```python
from build123d import *

# Parameters (mm, degrees)
SKETCH_1_W                  = 60
SKETCH_1_H                  = 45
SKETCH_1_R                  = 2.5
SKETCH_1_R_2                = 12
EXTRUDE_1_DEPTH             = 8
CHAMFER_1_SIZE              = 1
SKETCH_2_R                  = 4
CUT_EXTRUDE_1_DEPTH         = 6
SKETCH_3_R                  = 1.25
CUT_EXTRUDE_2_DEPTH         = 39.34383914
HOLE_WIZARD_2_D             = 6.2
HOLE_WIZARD_2_CSINK_D       = 13.2
HOLE_WIZARD_2_CSINK_ANGLE   = 90
HOLE_WIZARD_2_2_D           = 3.1
HOLE_WIZARD_2_2_CSINK_D     = 6.2
HOLE_WIZARD_2_2_CSINK_ANGLE = 90


with BuildPart() as part:
    # 草图1 → 凸台-拉伸1 (new body)
    with BuildSketch(Plane(origin=(0, 0, 0), x_dir=(1, 0, 0), z_dir=(0, 1, 0))):
        Rectangle(SKETCH_1_W, SKETCH_1_H)
        with Locations(Location((-20, -12.5, 0), (0, 0, 270))):
            Circle(SKETCH_1_R, mode=Mode.SUBTRACT)
        with Locations(Location((20, -12.5, 0), (0, 0, 90))):
            Circle(SKETCH_1_R, mode=Mode.SUBTRACT)
        with Locations(Location((0, -5, 0), (0, 0, 270))):
            Circle(SKETCH_1_R_2, mode=Mode.SUBTRACT)
    extrude(amount=EXTRUDE_1_DEPTH)

    # 倒角1
    chamfer_1_edges = [part.edges().sort_by_distance(p)[0] for p in [
        (0, 8, -22.5),
        (0, 0, -22.5),
    ]]
    chamfer(chamfer_1_edges, length=CHAMFER_1_SIZE)

    # 草图2 → 切除-拉伸1 (cut)
    with BuildSketch(Plane(origin=(0, 8, 0), x_dir=(1, 0, 0), z_dir=(0, 1, 0))):
        with Locations(Location((-19.5, 14.5, 0), (0, 0, 270))):
            Circle(SKETCH_2_R)
        with Locations(Location((19.5, 14.5, 0), (0, 0, 90))):
            Circle(SKETCH_2_R)
    extrude(amount=-CUT_EXTRUDE_1_DEPTH, mode=Mode.SUBTRACT)

    # 草图3 → 切除-拉伸2 (cut, through all)
    with BuildSketch(Plane(origin=(0, 0, 0), x_dir=(-1, 0, 0), z_dir=(0, -1, 0))):
        with Locations(Location((13, -18, 0), (0, 0, 90))):
            Circle(SKETCH_3_R)
        with Locations(Location((-13, -18, 0), (0, 0, 270))):
            Circle(SKETCH_3_R)
        with Locations(Location((13, 8, 0), (0, 0, 90))):
            Circle(SKETCH_3_R)
        with Locations(Location((-13, 8, 0), (0, 0, 270))):
            Circle(SKETCH_3_R)
    extrude(amount=-CUT_EXTRUDE_2_DEPTH, mode=Mode.SUBTRACT)

    # Hole Wizard 2 (through all)
    with Locations(Plane(origin=(20, 0, 12.5), x_dir=(0, 0, -1), z_dir=(0, -1, 0))):
        with Locations((0, 0), (0, -40)):
            CounterSinkHole(HOLE_WIZARD_2_D / 2, HOLE_WIZARD_2_CSINK_D / 2, counter_sink_angle=HOLE_WIZARD_2_CSINK_ANGLE)

    # Hole Wizard 2 2 (through all)
    with Locations(Plane(origin=(-13, 8, -8), x_dir=(0, 0, 1), z_dir=(0, 1, 0))):
        with Locations((0, 0), (26, 0), (26, 26), (0, 26)):
            CounterSinkHole(HOLE_WIZARD_2_2_D / 2, HOLE_WIZARD_2_2_CSINK_D / 2, counter_sink_angle=HOLE_WIZARD_2_2_CSINK_ANGLE)


solid = part.part
```
Geometry check sheet. Reference: the model listing, model coordinates, mm. A direction names the side the tool comes from. Round coordinates to 2 decimals unless told otherwise and drop trailing zeros. Write each loop counter-clockwise with the first axis right and the second up, starting at its lowest first coordinate (ties: lowest second). Pieces come first, ordered by that corner, then holes. Notation, with made-up numbers: (67.5, 25) -> (72.5, 25) arc R14 ccw to (72.5, 37) -> close; hole circle Ø3 at (-27.75, -34). An arc over 180 degrees is marked (long way). Put each result on its own line as item: value.
1) Cross-section at A-A, the plane z = -8. Enter the section's corners in (x, y).
Recorded:
outline: (-30, 0) -> (-14.55, 0) -> (-14.55, 6.45) -> (-16.1, 8) -> (-30, 8) -> close; (-11.45, 0) -> (11.45, 0) -> (11.45, 6.45) -> (9.9, 8) -> (-9.9, 8) -> (-11.45, 6.45) -> close; (14.55, 0) -> (30, 0) -> (30, 8) -> (16.1, 8) -> (14.55, 6.45) -> close
2) Thickness scan on probe 1 along Z at (x, y) = (-13, 3.25); probe 2 along X at (y, z) = (2.25, 18); probe 3 along X at (y, z) = (4.9, 12.5). Record the ranges inside material, lowest first. Write a range as from..to.
Recorded:
probe 1: z = -22.5..-9.55, -6.45..16.45, 19.55..22.5
probe 2: x = -30..-14.55, -11.45..11.45, 14.55..30
probe 3: x = -30..-23.1, -16.9..-9.37, 9.37..16.9, 23.1..30
3) Release check for a two-part mould opening along X. For faces 1 (the face through (-21.886, 5.781, 10.04)), 2 (the face through (0, 4, -22.5)) record: pulls with the +X half, pulls with the -X half, needs draft (parallel to the pull), parting line crosses it, or undercut.
Recorded:
face 1: undercut
face 2: needs draft
4) Access from +Z, -Z, +X, -X, +Y, -Y to the whole of each face (thin tool, end or side, straight path). Record for faces 3 (the face through (16.8, 5.04, -11.55)), 4 (the face through (-13.594, 3.18, 16.568)).
Recorded:
face 3: +Y
face 4: +Y, -Y
5) Cross-section at D-D, the plane z = -3. Enter the section's corners in (x, y), plus the area to 3 significant figures.
Recorded:
outline: (-30, 0) -> (-8.94, 0) -> (-8.94, 8) -> (-30, 8) -> close; (8.94, 0) -> (30, 0) -> (30, 8) -> (8.94, 8) -> close
area: 337 mm2
6) Cross-section at B-B, the plane x = 0. Enter the section's corners in (y, z), plus the area to 3 significant figures.
Recorded:
outline: (0, -21.5) -> (1, -22.5) -> (7, -22.5) -> (8, -21.5) -> (8, -7) -> (0, -7) -> close; (0, 17) -> (8, 17) -> (8, 22.5) -> (0, 22.5) -> close
area: 167 mm2
7) Depth check by flat-ended pin: P1, Ø5, axis at x = 12.5, z = 3.5, coming from the -Y side; P2, Ø19, axis at x = 0, z = 5, coming from the -Y side; P3, Ø4, axis at x = -13, z = -8, coming from the +Y side. Enter the tip coordinate at first touch or a pass-through.
Recorded:
P1: stops at y = 0
P2: passes through
P3: stops at y = 6.9
8) Cross-section at C-C, the plane y = 4.75. Give the number of separate pieces and of enclosed holes in the cut face, plus the area to 3 significant figures.
Recorded:
separate pieces: 1
enclosed holes: 9
area: 2,060 mm2
